Source: CAD feature listing. Evaluate the final solid. Frame: model axes, mm. Face numbers are marked on the shaded views. A direction names the side the tool comes from. Give positions to 0.01 mm unless a question says otherwise; leave off trailing zeros. Loops run counter-clockwise (first coordinate to the right, second up) from the corner with the lowest first, then second, coordinate; pieces in that order, holes last. Notation, with made-up numbers: (17, -19.75) -> (74, -19.75) arc R20 cw to (74, -9.75) -> close; hole circle Ø8 at (17.25, 49.5). An arc over 180 degrees is marked (long way). Answer as a JSON object with one key per item and string values. Group by question number.
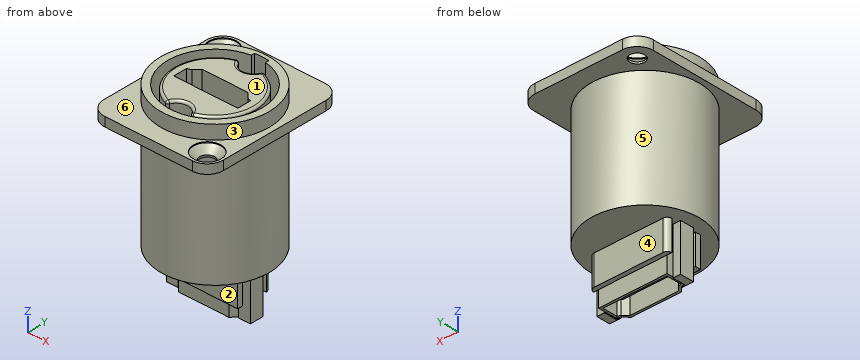
from build123d import *

# Parameters (mm, degrees)
ESQUISSE1_W                                 = 11.8
ESQUISSE1_H                                 = 25.5
ESQUISSE2_W                                 = 24.8
ESQUISSE2_H                                 = 27.3
BOSS_EXTRU_1_DEPTH                          = 2
ESQUISSE3_W                                 = 2
ESQUISSE3_H                                 = 27.3
BOSS_EXTRU_2_DEPTH                          = 1.2
BOSS_EXTRU_3_DEPTH                          = 10
ESQUISSE5_W                                 = 10
ESQUISSE5_H                                 = 1.115484429
ENL_V_MAT_EXTRU_1_DEPTH                     = 3.6
ESQUISSE6_W                                 = 10
ESQUISSE6_H                                 = 1.384515571
ENL_V_MAT_EXTRU_2_DEPTH                     = 1.65
ESQUISSE7_W                                 = 10
ESQUISSE7_H                                 = 1.384515571
ENL_V_MAT_EXTRU_3_DEPTH                     = 1.65
BOSS_EXTRU_4_DEPTH                          = 0.2
BOSS_EXTRU_5_DEPTH                          = 0.2
ESQUISSE10_W                                = 26
ESQUISSE10_H                                = 2
BOSS_EXTRU_6_DEPTH                          = 3.7
BOSS_EXTRU_7_START                          = 3
ESQUISSE11_R                                = 11.8
BOSS_EXTRU_7_DEPTH                          = 3
ENL_V_MAT_EXTRU_4_DEPTH                     = 14
BOSS_EXTRU_8_DEPTH                          = 13.5
ENL_V_MAT_EXTRU_5_DEPTH                     = 11
ESQUISSE15_W                                = 11
ESQUISSE15_H                                = 1
BOSS_EXTRU_9_DEPTH                          = 6.6
ENL_V_MAT_EXTRU_6_DEPTH                     = 12
ESQUISSE17_W                                = 11
ESQUISSE17_H                                = 1
BOSS_EXTRU_10_DEPTH                         = 9.6
D_POUILLE1_ANGLE                            = 20.013261752
D_POUILLE2_ANGLE                            = 20.013261752
D_POUILLE3_ANGLE                            = 20.013261752
D_POUILLE4_ANGLE                            = 20.013261752
D_POUILLE5_ANGLE                            = 43.186676481
D_POUILLE6_ANGLE                            = 43.186676481
D_POUILLE7_ANGLE                            = 43.186676481
FRAISAGE_POUR_VIS_T_TE_FRAIS_E_M31_AT_COUNT = 2
FRAISAGE_POUR_VIS_T_TE_FRAIS_E_M31_AT_PITCH = 30.61045573
NERVURE1_START                              = -8.5
NERVURE1_OUTLINE_W                          = 1
NERVURE1_OUTLINE_H                          = 6.5
NERVURE1_DEPTH                              = 17
NERVURE2_START                              = -8.5
NERVURE2_OUTLINE_W                          = 1.2
NERVURE2_OUTLINE_H                          = 6.5
NERVURE2_DEPTH                              = 17
CHANFREIN1_SIZE                             = 0.027978428
CHANFREIN1_SIZE2                            = 0.021236921
CHANFREIN2_SIZE                             = 0.027978428
CHANFREIN2_SIZE2                            = 0.021236921
CONG_1_R                                    = 0.5
CONG_2_R                                    = 1
CONG_3_R                                    = 3.5


# Read off the part's stored shape, not the designer's step: Nervure1, Nervure2
with BuildPart() as part:
    # Esquisse1 → Révolution1 (revolve)
    with BuildSketch(Plane.XZ, mode=Mode.PRIVATE) as r_volution1_sk:
        with Locations((5.9, -12.75)):
            Rectangle(ESQUISSE1_W, ESQUISSE1_H)
    revolve(r_volution1_sk.sketch.rotate(Axis((0, 0, 0), (0, 0, -1)), 180), axis=Axis((0, 0, 0), (0, 0, -1)))

    # Esquisse2 → Boss.-Extru.1 (add)
    with BuildSketch(Plane(origin=(0, 0, 0), x_dir=(-1, 0, 0), z_dir=(0, 0, -1))):
        with Locations((0.6, -1.85)):
            Rectangle(ESQUISSE2_W, ESQUISSE2_H)
    extrude(amount=-BOSS_EXTRU_1_DEPTH)

    # Esquisse3 → Boss.-Extru.2 (add)
    with BuildSketch(Plane(origin=(11.8, 0, 0), x_dir=(0, 0, -1), z_dir=(1, 0, 0))):
        with Locations((-1, -1.85)):
            Rectangle(ESQUISSE3_W, ESQUISSE3_H)
    extrude(amount=BOSS_EXTRU_2_DEPTH)

    # Esquisse4 → Boss.-Extru.3 (add)
    with BuildSketch(Plane(origin=(0, 0, -25.5), x_dir=(-1, 0, 0), z_dir=(0, 0, -1))):
        Polygon((-9.1, 2.85), (9.1, 2.85), (9.1, -2.65), (-5.5, -2.65), (-5.5, -1.534515571), (-9.1, -1.534515571), align=None)
    extrude(amount=BOSS_EXTRU_3_DEPTH)

    # Esquisse5 → Enlèv. mat.-Extru.1 (cut)
    with BuildSketch(Plane.ZY.offset(9.1)):
        with Locations((-30.5, -2.092257786)):
            Rectangle(ESQUISSE5_W, ESQUISSE5_H)
    extrude(amount=-ENL_V_MAT_EXTRU_1_DEPTH, mode=Mode.SUBTRACT)

    # Esquisse6 → Enlèv. mat.-Extru.2 (cut)
    with BuildSketch(Plane(origin=(9.1, 0, 0), x_dir=(0, 0, -1), z_dir=(1, 0, 0))):
        with Locations((30.5, 2.157742215)):
            Rectangle(ESQUISSE6_W, ESQUISSE6_H)
    extrude(amount=-ENL_V_MAT_EXTRU_2_DEPTH, mode=Mode.SUBTRACT)

    # Esquisse7 → Enlèv. mat.-Extru.3 (cut)
    with BuildSketch(Plane.ZY.offset(9.1)):
        with Locations((-30.5, 2.157742215)):
            Rectangle(ESQUISSE7_W, ESQUISSE7_H)
    extrude(amount=-ENL_V_MAT_EXTRU_3_DEPTH, mode=Mode.SUBTRACT)

    # Esquisse8 → Boss.-Extru.4 (add)
    with BuildSketch(Plane(origin=(0, 0, -35.5), x_dir=(-1, 0, 0), z_dir=(0, 0, -1))):
        Polygon((-6.575, -1.534515571), (-9.1, -1.534515571), (-9.1, 1.465484429), (-7.45, 1.465484429), (-7.45, -1.215812238), align=None)
    extrude(amount=BOSS_EXTRU_4_DEPTH)

    # Esquisse9 → Boss.-Extru.5 (add)
    with BuildSketch(Plane(origin=(0, 0, -35.5), x_dir=(-1, 0, 0), z_dir=(0, 0, -1))):
        Polygon((6.575, -1.534515571), (7.45, -1.215812238), (7.45, 1.465484429), (9.1, 1.465484429), (9.1, -1.534515571), align=None)
    extrude(amount=BOSS_EXTRU_5_DEPTH)

    # Esquisse10 → Boss.-Extru.6 (add)
    with BuildSketch(Plane(origin=(0, 11.8, 0), x_dir=(-1, 0, 0), z_dir=(0, 1, 0))):
        with Locations((0, 1)):
            Rectangle(ESQUISSE10_W, ESQUISSE10_H)
    extrude(amount=BOSS_EXTRU_6_DEPTH)

    # Esquisse11 → Boss.-Extru.7 (add)
    with BuildSketch(Plane.XY.offset(2).offset(BOSS_EXTRU_7_START)):
        with Locations(Location((0, 0, 0), (0, 0, 180))):
            Circle(ESQUISSE11_R)
    extrude(amount=-BOSS_EXTRU_7_DEPTH)

    # Esquisse12 → Enlèv. mat.-Extru.4 (cut)
    with BuildSketch(Plane.XY.offset(5)):
        with BuildLine():
            Line((1.55, 10.132127121), (1.55, 10.890247931))
            ThreePointArc((1.55, 10.890247931), (0, 11), (-1.55, 10.890247931))
            Line((-1.55, 10.890247931), (-1.55, 10.132127121))
            ThreePointArc((-1.55, 10.132127121), (0, -10.25), (1.55, 10.132127121))
        make_face()
    extrude(amount=-ENL_V_MAT_EXTRU_4_DEPTH, mode=Mode.SUBTRACT)

    # Esquisse13 → Boss.-Extru.8 (add)
    with BuildSketch(Plane.XY.offset(-9)):
        with BuildLine():
            ThreePointArc((2.525486644, -8.482005495), (0, -6.5), (-2.525486644, -8.482005495))
            ThreePointArc((-2.525486644, -8.482005495), (-8.85, 0), (-2.525486644, 8.482005495))
            ThreePointArc((-2.525486644, 8.482005495), (0, 6.5), (2.525486644, 8.482005495))
            ThreePointArc((2.525486644, 8.482005495), (8.85, 0), (2.525486644, -8.482005495))
        make_face()
    extrude(amount=BOSS_EXTRU_8_DEPTH)

    # Esquisse14 → Enlèv. mat.-Extru.5 (cut)
    with BuildSketch(Plane.XY.offset(4.5)):
        Polygon((5, 0.85), (5, 2.35), (-5, 2.35), (-5, 0.85), (-6.95, 0.85), (-6.95, -2.15), (6.95, -2.15), (6.95, 0.85), align=None)
    extrude(amount=-ENL_V_MAT_EXTRU_5_DEPTH, mode=Mode.SUBTRACT)

    # Esquisse15 → Boss.-Extru.9 (add)
    with BuildSketch(Plane.XY.offset(-6.5)):
        with Locations((0, 0.05)):
            Rectangle(ESQUISSE15_W, ESQUISSE15_H)
    extrude(amount=BOSS_EXTRU_9_DEPTH)

    # Esquisse16 → Enlèv. mat.-Extru.6 (cut)
    with BuildSketch(Plane(origin=(0, 0, -35.5), x_dir=(-1, 0, 0), z_dir=(0, 0, -1))):
        Polygon((5.283561654, -2.15), (5.283561654, -0.865794698), (6.95, -0.865794698), (6.95, 2.35), (-6.95, 2.35), (-6.95, -0.865794698), (-5.283561654, -0.865794698), (-5.283561654, -2.15), align=None)
    extrude(amount=-ENL_V_MAT_EXTRU_6_DEPTH, mode=Mode.SUBTRACT)

    # Esquisse17 → Boss.-Extru.10 (add)
    with BuildSketch(Plane(origin=(0, 0, -23.5), x_dir=(-1, 0, 0), z_dir=(0, 0, -1))):
        with Locations((0, -0.15)):
            Rectangle(ESQUISSE17_W, ESQUISSE17_H)
    extrude(amount=BOSS_EXTRU_10_DEPTH)

    # Dépouille1
    d_pouille1_faces = [part.faces().sort_by_distance(p)[0] for p in [
        (-6.116780827, -0.865794698, -29.5),
    ]]
    draft(d_pouille1_faces, Plane(origin=(-6.95, -0.865794698, -23.5), x_dir=(0, 1, 0), z_dir=(1, 0, 0)), D_POUILLE1_ANGLE)

    # Dépouille2
    d_pouille2_faces = [part.faces().sort_by_distance(p)[0] for p in [
        (6.116780827, -0.865794698, -29.5),
    ]]
    draft(d_pouille2_faces, Plane(origin=(6.95, 2.35, -23.5), x_dir=(0, -1, 0), z_dir=(-1, 0, 0)), D_POUILLE2_ANGLE)

    # Dépouille3
    d_pouille3_faces = [part.faces().sort_by_distance(p)[0] for p in [
        (-5.975, 0.85, -1),
    ]]
    draft(d_pouille3_faces, Plane(origin=(-6.95, 0.85, -6.5), x_dir=(0, 1, 0), z_dir=(1, 0, 0)), D_POUILLE3_ANGLE)

    # Dépouille4
    d_pouille4_faces = [part.faces().sort_by_distance(p)[0] for p in [
        (5.975, 0.85, -1),
    ]]
    draft(d_pouille4_faces, Plane(origin=(6.95, -2.15, -6.5), x_dir=(0, 0, -1), z_dir=(-1, 0, 0)), D_POUILLE4_ANGLE)

    # Dépouille5
    d_pouille5_faces = [part.faces().sort_by_distance(p)[0] for p in [
        (5.5, -2.092257785, -30.5),
        (-5.5, -2.092257785, -30.5),
    ]]
    draft(d_pouille5_faces, Plane(origin=(-9.1, -2.65, -35.5), x_dir=(-1, 0, 0), z_dir=(0, -1, 0)), D_POUILLE5_ANGLE)

    # Dépouille6
    d_pouille6_faces = [part.faces().sort_by_distance(p)[0] for p in [
        (-5.283561654, -1.811382752, -29.5),
        (5.283561654, -1.811382752, -29.5),
    ]]
    draft(d_pouille6_faces, Plane(origin=(5.283561654, -2.15, -23.5), x_dir=(1, 0, 0), z_dir=(0, 1, 0)), D_POUILLE6_ANGLE)

    # Dépouille7
    d_pouille7_faces = [part.faces().sort_by_distance(p)[0] for p in [
        (-5, 1.955126571, -1),
        (5, 1.955126571, -1),
    ]]
    draft(d_pouille7_faces, Plane(origin=(5, 2.35, -6.5), x_dir=(-1, 0, 0), z_dir=(0, -1, 0)), D_POUILLE7_ANGLE)

    # Esquisse18 → Fraisage pour vis à tête fraisée M31 (revolve, cut)
    with BuildSketch(Plane(origin=(-9.5, 12, 2), x_dir=(0, -1, 0), z_dir=(1, 0, 0))):
        Polygon((0, 0), (0, 37.700025), (1.6, 37.700025), (1.6, 1.599995685), (3, 0.19999191), (3, 0), align=None)
    fraisage_pour_vis_t_te_frais_e_m31 = revolve(axis=Axis((-9.5, 12, 8.35), (0, 0, -1)), mode=Mode.SUBTRACT)

    # Fraisage pour vis à tête fraisée M31 at: Fraisage pour vis à tête fraisée M31 ×2
    with Locations(*[Vector(0.6207029443655612, -0.7840458244617614, 0) * (i * FRAISAGE_POUR_VIS_T_TE_FRAIS_E_M31_AT_PITCH) for i in range(1, FRAISAGE_POUR_VIS_T_TE_FRAIS_E_M31_AT_COUNT)]):
        add(fraisage_pour_vis_t_te_frais_e_m31, mode=Mode.SUBTRACT)

    # Nervure1 outline → Nervure1 (add)
    with BuildSketch(Plane(origin=(0, 0, 0), x_dir=(0, -1, 0), z_dir=(-1, 0, 0)).offset(NERVURE1_START)):
        with Locations((-3.35, -28.75)):
            Rectangle(NERVURE1_OUTLINE_W, NERVURE1_OUTLINE_H)
    extrude(amount=NERVURE1_DEPTH)

    # Nervure2 outline → Nervure2 (add)
    with BuildSketch(Plane(origin=(0, 0, 0), x_dir=(0, -1, 0), z_dir=(-1, 0, 0)).offset(NERVURE2_START)):
        with Locations((3.25, -28.75)):
            Rectangle(NERVURE2_OUTLINE_W, NERVURE2_OUTLINE_H)
    extrude(amount=NERVURE2_DEPTH)

    # Chanfrein1
    chanfrein1_edges = [part.edges().sort_by_distance(p)[0] for p in [
        (6.547021572, -1.534515571, -30.5),
    ]]
    chanfrein1_side = [part.faces().sort_by_distance(p)[0] for p in [
        (7.823782137, -1.534515571, -30.598925344),
    ]]
    chamfer(chanfrein1_edges, length=CHANFREIN1_SIZE, length2=CHANFREIN1_SIZE2, reference=chanfrein1_side[0])

    # Chanfrein2
    chanfrein2_edges = [part.edges().sort_by_distance(p)[0] for p in [
        (-6.547021572, -1.534515571, -30.5),
    ]]
    chanfrein2_side = [part.faces().sort_by_distance(p)[0] for p in [
        (-7.823782137, -1.534515571, -30.598925344),
    ]]
    chamfer(chanfrein2_edges, length=CHANFREIN2_SIZE, length2=CHANFREIN2_SIZE2, reference=chanfrein2_side[0])

    # Congé1
    cong_1_edges = [part.edges().sort_by_distance(p)[0] for p in [
        (2.525486644, -8.482005495, -2.25),
        (2.525486644, 8.482005495, -2.25),
        (-2.525486644, 8.482005495, -2.25),
        (-2.525486644, -8.482005495, -2.25),
        (8.85, 0, 4.5),
        (0, 6.5, 4.5),
        (-8.85, 0, 4.5),
        (0, -6.5, 4.5),
    ]]
    fillet(cong_1_edges, radius=CONG_1_R)

    # Congé2
    cong_2_edges = [part.edges().sort_by_distance(p)[0] for p in [
        (8.5, 3.85, -28.75),
        (-8.5, 3.85, -28.75),
    ]]
    fillet(cong_2_edges, radius=CONG_2_R - 0.0001)  # a hair under: the kernel refuses the full size

    # Congé3
    cong_3_edges = [part.edges().sort_by_distance(p)[0] for p in [
        (-13, -15.5, 1),
        (13, 15.5, 1),
        (-13, 15.5, 1),
        (13, -15.5, 1),
    ]]
    fillet(cong_3_edges, radius=CONG_3_R)


solid = part.part
(1) Section query C-C on z = -12.5. Return the cut outline in (x, y).
(2) Material intervals for line 1 (Y direction, x = -2.5, z = -30.5); line 2 (Y direction, x = 9.5, z = 0.3); line 3 (X direction, y = -12, z = 0.3), sorted ascending. Write a range as from..to.
(3) Mould query, pull axis X, two halves, no side actions, for the marked faces 1, 2 and 3. Classes: pulls with the +X half, pulls with the -X half, needs draft (parallel to the pull), parting line crosses it, or undercut.
(4) Section query A-A on z = -29. State how many separate pieces and enclosed holes the cut face has, plus the area to 3 significant figures.
(5) First-contact query: pin 1 (5 mm diameter, centred on y = 3.5, z = -18, fed in from +X); pin 2 (2 mm diameter, centred on x = 8, z = -31.5, fed in from -Y); pin 3 (2.5 mm diameter, centred on y = 0.5, z = -32.5, fed in from -X). Flat tips, straight axial feed; report the tip coordinate or a pass-through.
(6) Access query for the marked faces 4, 5 and 6. Directions: +Z, -Z, +X, -X, +Y, -Y. A direction counts if a zero-diameter tool reaches every point of the face in a straight line with its end or side. Return the directions, or none.
Result:
{
 "1": {"outline": "circle Ø23.6 at (0, 0)"},
 "2": {"line 1": "-3.85..-2.15, -0.65..0.35, 2.35..3.85", "line 2": "-15.5..-13.6, -10.4..-3.85, 3.85..15.5", "line 3": "-13..7.9, 11.1..13"},
 "3": {"face 1": "undercut", "face 2": "needs draft", "face 3": "parting line crosses it"},
 "4": {"separate pieces": "2", "enclosed holes": "1", "area": "76.7 mm²"},
 "5": {"pin 1": "x = 11.76", "pin 2": "y = -3.85", "pin 3": "x = -9.1"},
 "6": {"face 4": "-Z, +X, -X, +Y", "face 5": "-Z", "face 6": "+Z"}
}
